Here's how the part is built. I have some questions about the finished solid (model axes, mm). Face numbers are marked on the shaded views. A direction names the side the tool comes from. Coordinates: 2 decimals unless noted, no trailing zeros. Write each loop counter-clockwise with the first axis right and the second up, starting at its lowest first coordinate (ties: lowest second). Pieces come first, ordered by that corner, then holes. Notation, with made-up numbers: (18.5, 5) -> (36.5, 5) arc R24 ccw to (36.5, 31) -> close; hole circle Ø9 at (31.5, -16). An arc over 180 degrees is marked (long way). Put each result on its own line as item: value.
```python
from build123d import *

# Parameters (mm, degrees)
SALIENTE_EXTRUIR1_DEPTH = 18.5
CORTAR_EXTRUIR1_DEPTH   = 53.5
CROQUIS4_R              = 4
CROQUIS4_W              = 2.6
CROQUIS4_H              = 10
SALIENTE_EXTRUIR3_DEPTH = 3


with BuildPart() as part:
    # Croquis1 → Saliente-Extruir1 (new, symmetric)
    with BuildSketch(Plane.XY):
        with BuildLine():
            Line((-34, 44.6), (-34, -31.4))
            ThreePointArc((-34, -31.4), (0, -25), (34, -31.4))
            Line((34, -31.4), (34, 31.6))
            Line((34, 31.6), (22.75, 33.6))
            Line((22.75, 33.6), (17.75, 26.215384615))
            Line((17.75, 26.215384615), (17.75, 0))
            ThreePointArc((17.75, 0), (0, -17.75), (-17.75, 0))
            Line((-17.75, 0), (-18.75, 44.6))
            Line((-18.75, 44.6), (-34, 44.6))
        make_face()
    extrude(amount=SALIENTE_EXTRUIR1_DEPTH, both=True)

    # Croquis2 → Cortar-Extruir1 (cut, symmetric)
    with BuildSketch(Plane(origin=(0, 0, 0), x_dir=(1, 0, 0), z_dir=(0, 1, 0))):
        Polygon((-18.75, -15.5), (-31, -15.5), (-31, 15.5), (-18.75, 15.5), (-17.75, 15.5), (17.75, 15.5), (22.75, 15.5), (31, 15.5), (31, -15.5), (22.75, -15.5), (17.75, -15.5), (-17.75, -15.5), align=None)
    extrude(amount=CORTAR_EXTRUIR1_DEPTH, both=True, mode=Mode.SUBTRACT)

    # Croquis3 → Revolución1 (revolve)
    with BuildSketch(Plane.XY, mode=Mode.PRIVATE) as revoluci_n1_sk:
        Polygon((-34, 17.6), (-34, 3.6), (-37, 3.6), (-37, 10.3), (-41, 10.3), (-41, 4.9), (-45, 4.9), (-45, 17.6), align=None)
    revolve(revoluci_n1_sk.sketch.rotate(Axis((19.47822933, 17.6, 0), (-1, 0, 0)), 180), axis=Axis((19.47822933, 17.6, 0), (-1, 0, 0)))

    # Croquis4 → Saliente-Extruir3 (add)
    with BuildSketch(Plane.XY.offset(18.5)):
        with Locations((-25.5, 37.27)):
            Circle(CROQUIS4_R)
        with Locations((-32, 32.27)):
            Rectangle(CROQUIS4_W, CROQUIS4_H)
    extrude(amount=SALIENTE_EXTRUIR3_DEPTH)


solid = part.part
```
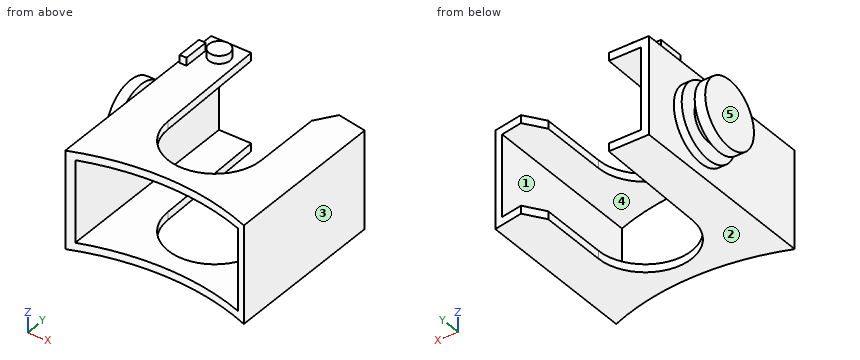
Item 1: Imagine slicing it at A-A on x = 0. Write out the boundary of the cut face in (y, z), then the cut area to 3 significant figures.
Output:
outline: (-25, -18.5) -> (-17.75, -18.5) -> (-17.75, -15.5) -> (-25, -15.5) -> close; (-25, 15.5) -> (-17.75, 15.5) -> (-17.75, 18.5) -> (-25, 18.5) -> close
area: 43.5 mm²
Item 2: If we mould it in two halves opening along Z, with no side actions, what happens to the marked faces 1, 2 and 3? For each: released by +Z, released by -Z, zero draft, split by the parting line, or undercut.
Output:
face 1: undercut
face 2: released by -Z
face 3: zero draft
Item 3: Imagine slicing it at D-D on y = 35. Write out the boundary of the cut face in (x, z).
Output:
outline: (-34, -18.5) -> (-18.53, -18.5) -> (-18.53, -15.5) -> (-31, -15.5) -> (-31, 15.5) -> (-18.53, 15.5) -> (-18.53, 18.5) -> (-22.21, 18.5) -> (-22.21, 21.5) -> (-28.79, 21.5) -> (-28.79, 18.5) -> (-30.7, 18.5) -> (-30.7, 21.5) -> (-33.3, 21.5) -> (-33.3, 18.5) -> (-34, 18.5) -> close
Item 4: Imagine slicing it at B-B on z = 0. Write out the boundary of the cut face in (x, y) (1 decimal).
Output:
outline: (-45, 4.9) -> (-41, 4.9) -> (-41, 10.3) -> (-37, 10.3) -> (-37, 3.6) -> (-34, 3.6) -> (-34, -31.4) arc R93.5 cw to (-31, -30.3) -> (-31, 44.6) -> (-34, 44.6) -> (-34, 31.6) -> (-37, 31.6) -> (-37, 24.9) -> (-41, 24.9) -> (-41, 30.3) -> (-45, 30.3) -> close; (31, -30.3) arc R93.5 cw to (34, -31.4) -> (34, 31.6) -> (31, 32.1) -> close
Item 5: For P1, Ø6, axis at y = -20.5, z = -2.5, coming from the -X side; P2, Ø6, axis at x = 16, y = 33, coming from the -Z side; P3, Ø2.5, axis at y = 31, z = 20, coming from the +X side; P4, Ø0.8, axis at x = -31.5, z = 20, coming from the -Y side, each with a flat end and sliding along its axis, tell me the tip position at first contact or that it passes through.
Output:
P1: stops at x = -34
P2: passes through
P3: stops at x = -30.7
P4: stops at y = 27.27
Item 6: Imagine slicing it at C-C on y = 23. Write out the boundary of the cut face in (x, z).
Output:
outline: (-45, -11.49) -> (-41, -11.49) -> (-41, -4.91) -> (-37, -4.91) -> (-37, -12.92) -> (-34, -12.92) -> (-34, -18.5) -> (-18.27, -18.5) -> (-18.27, -15.5) -> (-31, -15.5) -> (-31, 15.5) -> (-18.27, 15.5) -> (-18.27, 18.5) -> (-34, 18.5) -> (-34, 12.92) -> (-37, 12.92) -> (-37, 4.91) -> (-41, 4.91) -> (-41, 11.49) -> (-45, 11.49) -> close; (17.75, -18.5) -> (34, -18.5) -> (34, 18.5) -> (17.75, 18.5) -> (17.75, 15.5) -> (31, 15.5) -> (31, -15.5) -> (17.75, -15.5) -> close
Item 7: Please list where these lines run through material, in increasing order: line 1 along X through (y, z) = (-18, -10); line 2 along Z through (x, y) = (-10, -19.5); line 3 along X through (y, z) = (29.5, 6.5). Write a range as from..to.
Output:
line 1: x = -34..-31, 31..34
line 2: z = -18.5..-15.5, 15.5..18.5
line 3: x = -37..-31, 31..34
Item 8: Which directions (+Z, -Z, +X, -X, +Y, -Y) give clear straight access to the entire face, cutting with the end or side of a thin tool? Please do the marked faces 4 and 5.
Output:
face 4: +Y, -Y
face 5: +Z, -Z, -X, +Y, -Y
